Build history of the part. All positions in model axes, mm. Face numbers are marked on the shaded views. A direction names the side the tool comes from. Round coordinates to 2 decimals unless told otherwise and drop trailing zeros. Write each loop counter-clockwise with the first axis right and the second up, starting at its lowest first coordinate (ties: lowest second). Pieces come first, ordered by that corner, then holes.
1) Saw through at A-A (x = 98). Write the cut outline in (y, z), plus the area to 3 significant figures.
2) Saw through at B-B (y = -515.5). Write the cut outline in (x, z), plus the area to 3 significant figures.
3) Flat gauge pins, fed straight in: pin 1 (4 mm diameter, centred on x = -842.5, z = 62, fed in from -Y); pin 2 (1.5 mm diameter, centred on x = 196, y = -178, fed in from -Z). Where does each tip first touch, or does it go through?
4) Which spindle directions (+Z, -Z, +X, -X, +Y, -Y) get a long thin tool onto all of the face, cutting with end or side? Do the marked faces 1, 2 and 3. Say none if no direction does.
5) Wall check: probe 1 along X at (y, z) = (-438, 60); probe 2 along X at (y, z) = (478.5, 134.5); probe 3 along X at (y, z) = (-403, 52.5). Give the ranges that are in metal, low to high.
6) Saw through at C-C (y = 243). Write the cut outline in (x, z).
7) Pull direction X, two halves, no side cores. Call the marked faces 4, 5 and 6: +X half, -X half, draft (parallel to the pull), parting line (faces both ways), or undercut.
8) Saw through at D-D (x = -363). Write the cut outline in (y, z), plus the area to 3 significant figures.
from build123d import *

# Parameters (mm, degrees)
F0_R     = 46.99
F0_R_2   = 46.986706
F0_R_3   = 294.64
F1_DEPTH = 184.15


with BuildPart() as f1:
    # F0 (on Top) → F1 (new body)
    with BuildSketch(Plane.XY):
        with BuildLine():
            ThreePointArc((564.590297, 572.830329), (557.150809, 590.790842), (539.190297, 598.230329))
            Line((539.190297, 598.230329), (-854.324554, 598.230329))
            ThreePointArc((-854.324554, 598.230329), (-857.294719, 597.391413), (-859.38711, 595.122589))
            Line((-859.38711, 595.122589), (-1351.950452, -375.304965))
            Line((-1351.950452, -375.304965), (-1351.950452, -603.904965))
            ThreePointArc((-1351.950452, -603.904965), (-1344.510965, -621.865477), (-1326.550452, -629.304965))
            Line((-1326.550452, -629.304965), (-991.270452, -629.304965))
            Line((-991.270452, -629.304965), (-991.270452, -484.524965))
            Line((-991.270452, -484.524965), (-1021.750452, -484.524965))
            Line((-1021.750452, -484.524965), (-1021.750452, -408.324965))
            Line((-1021.750452, -408.324965), (-991.270452, -408.324965))
            Line((-991.270452, -408.324965), (-991.270452, -281.324965))
            Line((-991.270452, -281.324965), (-905.926452, -281.324965))
            Line((-905.926452, -281.324965), (-905.926452, -408.324965))
            Line((-905.926452, -408.324965), (-875.446452, -408.324965))
            Line((-875.446452, -408.324965), (-875.446452, -484.524965))
            Line((-875.446452, -484.524965), (-905.926452, -484.524965))
            Line((-905.926452, -484.524965), (-905.926452, -629.304965))
            Line((-905.926452, -629.304965), (-829.139571, -629.304965))
            ThreePointArc((-829.139571, -629.304965), (-811.179058, -636.744453), (-803.739571, -654.704965))
            Line((-803.739571, -654.704965), (-803.739571, -774.084965))
            ThreePointArc((-803.739571, -774.084965), (-796.300083, -792.045477), (-778.339571, -799.484965))
            Line((-778.339571, -799.484965), (-450.679571, -799.484965))
            ThreePointArc((-450.679571, -799.484965), (-432.719058, -792.045477), (-425.279571, -774.084965))
            Line((-425.279571, -774.084965), (-425.279571, -654.704965))
            ThreePointArc((-425.279571, -654.704965), (-417.840083, -636.744453), (-399.879571, -629.304965))
            Line((-399.879571, -629.304965), (-78.648547, -629.304965))
            Line((-78.648547, -629.304965), (-78.648547, -484.524965))
            Line((-78.648547, -484.524965), (-109.128547, -484.524965))
            Line((-109.128547, -484.524965), (-109.128547, -408.324965))
            Line((-109.128547, -408.324965), (-78.648547, -408.324965))
            Line((-78.648547, -408.324965), (-78.648547, -281.324965))
            Line((-78.648547, -281.324965), (6.695453, -281.324965))
            Line((6.695453, -281.324965), (6.695453, -408.324965))
            Line((6.695453, -408.324965), (37.175453, -408.324965))
            Line((37.175453, -408.324965), (37.175453, -484.524965))
            Line((37.175453, -484.524965), (6.695453, -484.524965))
            Line((6.695453, -484.524965), (6.695453, -629.304965))
            Line((6.695453, -629.304965), (159.095453, -629.304965))
            ThreePointArc((159.095453, -629.304965), (177.055965, -636.744453), (184.495453, -654.704965))
            Line((184.495453, -654.704965), (184.495453, -774.084965))
            ThreePointArc((184.495453, -774.084965), (191.934941, -792.045477), (209.895453, -799.484965))
            Line((209.895453, -799.484965), (335.990297, -799.484965))
            ThreePointArc((335.990297, -799.484965), (497.634907, -732.529575), (564.590297, -570.884965))
            Line((564.590297, -570.884965), (564.590297, 572.830329))
        make_face()
        with Locations((-367.995667, -423.121417)):
            Circle(F0_R, mode=Mode.SUBTRACT)
        with Locations((419.586441, -423.096056)):
            Circle(F0_R_2, mode=Mode.SUBTRACT)
        with Locations((62.190297, 123.390329)):
            Circle(F0_R_3, mode=Mode.SUBTRACT)
        with Locations((-367.589703, 460.816329)):
            Circle(F0_R, mode=Mode.SUBTRACT)
        with Locations((422.350297, 460.816329)):
            Circle(F0_R, mode=Mode.SUBTRACT)
    extrude(amount=F1_DEPTH)


solid = f1.part
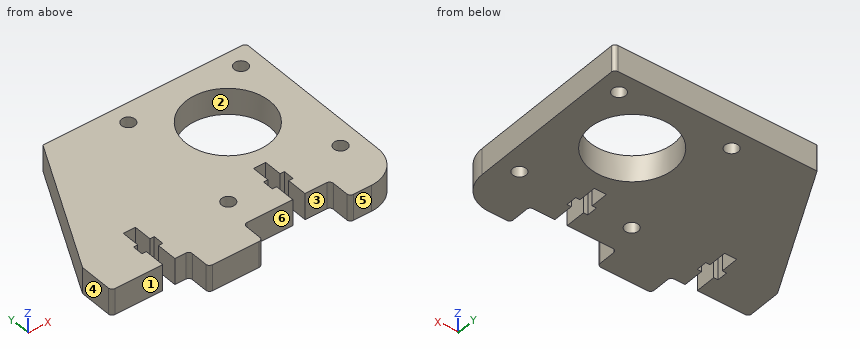
Evaluation:
1. outline: (-629.3, 0) - (-169.07, 0) - (-169.07, 184.15) - (-629.3, 184.15) - close; (415.85, 0) - (598.23, 0) - (598.23, 184.15) - (415.85, 184.15) - close
1. area: 118,000 mm2
2. outline: (-1351.95, 0) - (-991.27, 0) - (-991.27, 184.15) - (-1351.95, 184.15) - close; (-905.93, 0) - (-78.65, 0) - (-78.65, 184.15) - (-905.93, 184.15) - close; (6.7, 0) - (564.59, 0) - (564.59, 184.15) - (6.7, 184.15) - close
2. area: 321,000 mm2
3. pin 1: stops at y = -629.3
3. pin 2: stops at z = 0
4. face 1: +Z, -Z, -X, -Y
4. face 2: +Z, -Z
4. face 3: +Z, -Z, -Y
5. probe 1: x = -1351.95 to -1021.75, -875.45 to -412.57, -323.42 to -109.13, 37.18 to 375.03, 464.15 to 564.59
5. probe 2: x = -918.58 to -411.13, -324.05 to 378.81, 465.89 to 564.59
5. probe 3: x = -1351.95 to -991.27, -905.93 to -410.46, -325.53 to -78.65, 6.7 to 377.11, 462.06 to 564.59
6. outline: (-1038.12, 0) - (-207.08, 0) - (-207.08, 184.15) - (-1038.12, 184.15) - close; (331.46, 0) - (564.59, 0) - (564.59, 184.15) - (331.46, 184.15) - close
7. face 4: -X half
7. face 5: draft
7. face 6: undercut
8. outline: (-629.3, 0) - (-469.85, 0) - (-469.85, 184.15) - (-629.3, 184.15) - close; (-376.4, 0) - (414.05, 0) - (414.05, 184.15) - (-376.4, 184.15) - close; (507.58, 0) - (598.23, 0) - (598.23, 184.15) - (507.58, 184.15) - close
8. area: 192,000 mm2
